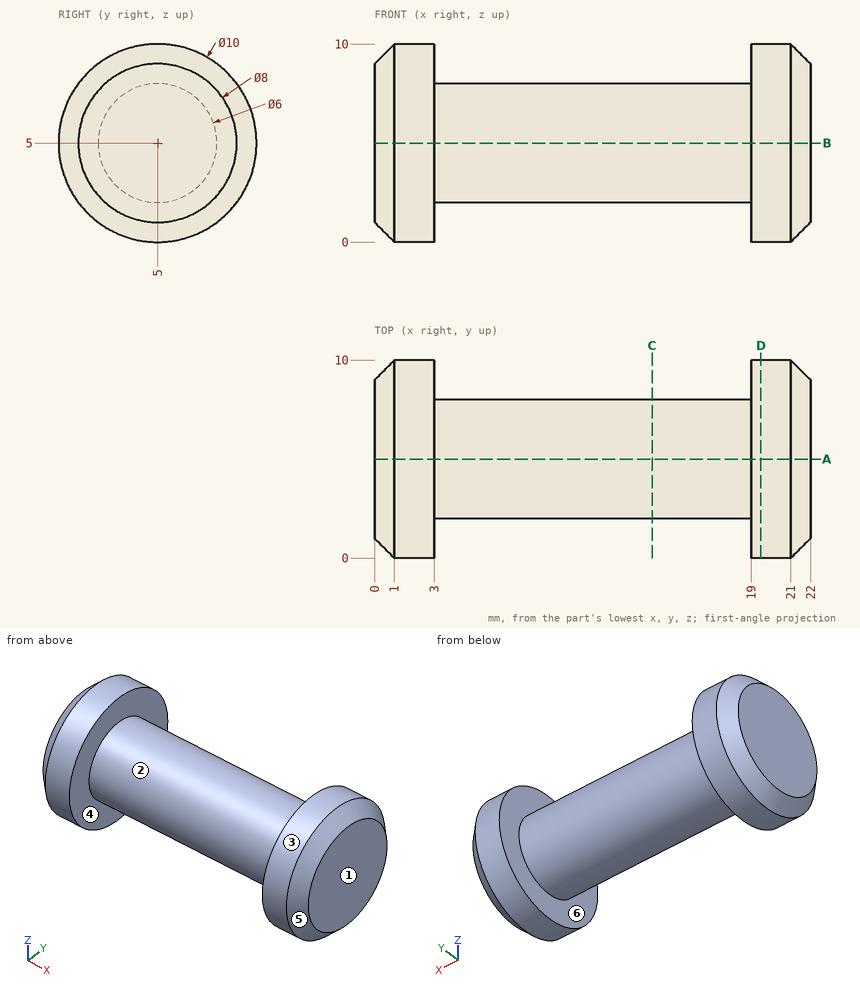
For this review, use the dimensioned drawing (mm, ordinates from the lowest corner) and the shaded views. A direction names the side the tool comes from. Round coordinates to 2 decimals unless told otherwise and drop trailing zeros. Order: outer loops, then holes, each group sorted by start corner. A loop starts at its lowest first (then second) coordinate and runs counter-clockwise, first axis right, second up. Notation, with made-up numbers: (22, -17) -> (44, -17) arc R24 cw to (44, -6) -> close; hole circle Ø10 at (10, 26). An arc over 180 degrees is marked (long way). Write item = value, one per line. Start each with the question number.
Item 1: Mouldability with a two-part tool opening along X and no side actions: class the marked faces 1, 2, 3 and 4 as released by +X, released by -X, zero draft, split by the parting line, or undercut.
Item 2: For the marked faces 5 and 6, list the 3-axis set-ups (+Z, -Z, +X, -X, +Y, -Y) from which the entire face can be reached by the end or side of a thin tool; tool diameter is ignored.
Item 3: Consider section D-D on x = 19.5. Write out the cut boundary in (y, z), plus the area to 3 significant figures.
Item 4: Clearance check with flat-ended pins moving along their axes: pin 1 Ø2 at (x, z) = (7.5, 6) entering from -Y; pin 2 Ø6 at (x, y) = (14.5, 8) entering from -Z; pin 3 Ø6 at (y, z) = (7.5, 1) entering from -X. State where each tip first meets the part, or that it passes through.
Item 5: For line 1 along Y through (x, z) = (12.75, 5); line 2 along X through (y, z) = (8.5, 8.5); line 3 along Z through (x, y) = (12.75, 6.25), list the stretches that pass through material, from the lowest coordinate up.
Item 6: Consider section A-A on y = 5. Write out the cut boundary in (x, z), plus the area to 3 significant figures.
Item 7: Consider section C-C on x = 14. Write out the cut boundary in (y, z).
Conclusion:
q1.face_1 = released by +X
q1.face_2 = undercut
q1.face_3 = zero draft
q1.face_4 = undercut
q2.face_5 = +X
q2.face_6 = none
q3.outline = circle Ø10 at (5, 5)
q3.area = 78.5 mm2
q4.pin_1 = 2
q4.pin_2 = 2
q4.pin_3 = 0
q5.line_1 = 2 to 8
q5.line_2 = 0.95 to 3, 19 to 21.05
q5.line_3 = 2.27 to 7.73
q6.outline = (0, 1) -> (1, 0) -> (3, 0) -> (3, 2) -> (19, 2) -> (19, 0) -> (21, 0) -> (22, 1) -> (22, 9) -> (21, 10) -> (19, 10) -> (19, 8) -> (3, 8) -> (3, 10) -> (1, 10) -> (0, 9) -> close
q6.area = 154 mm2
q7.outline = circle Ø6 at (5, 5)
